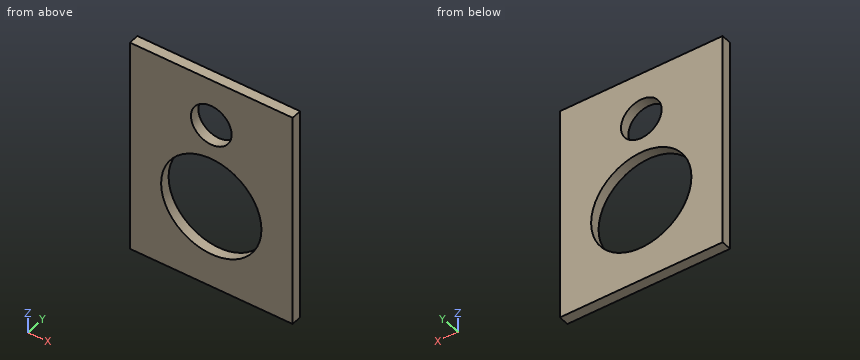
from build123d import *

# Parameters (mm, degrees)
F0_W     = 300
F0_H     = 400
F1_DEPTH = 19
F2_R     = 37.5
F2_R_2   = 92.5
F3_DEPTH = 19


with BuildPart() as f1:
    # F0 (on Front) → F1 (new body)
    with BuildSketch(Plane.XZ):
        with Locations((-9.787694, 40.103535)):
            Rectangle(F0_W, F0_H)
    extrude(amount=F1_DEPTH)

    # F2 (on face) → F3 (cut)
    with BuildSketch(Plane.XZ.offset(19)):
        with Locations((-9.787694, 152.603535)):
            Circle(F2_R)
        with Locations((-9.787694, -4.896465)):
            Circle(F2_R_2)
    extrude(amount=-F3_DEPTH, mode=Mode.SUBTRACT)


solid = f1.part
CAD build for the part. Positions are in the model's coordinates, mm. Give positions to 0.01 mm unless a question says otherwise; leave off trailing zeros. Order: outer loops, then holes, each group sorted by start corner. A loop starts at its lowest first (then second) coordinate and runs counter-clockwise, first axis right, second up. Notation, with made-up numbers: (0.25, 57) -> (55.25, 57) arc R20 cw to (55.25, 82) -> close; hole circle Ø9 at (88, 27.5). An arc over 180 degrees is marked (long way). Return JSON: item names as keys, results as strings.
Q1. Saw through at A-A (x = 46). Write the cut outline in (y, z).
Working result:
{"outline": "(-19, -159.9) -> (0, -159.9) -> (0, -78.68) -> (-19, -78.68) -> close; (-19, 68.89) -> (0, 68.89) -> (0, 240.1) -> (-19, 240.1) -> close"}
Q2. Saw through at C-C (y = -15). Write the cut outline in (x, z), then the cut area to 3 significant figures.
Working result:
{"outline": "(-159.79, -159.9) -> (140.21, -159.9) -> (140.21, 240.1) -> (-159.79, 240.1) -> close; hole circle Ø185 at (-9.79, -4.9); hole circle Ø75 at (-9.79, 152.6)", "area": "88,700 mm²"}
Q3. Drill centre lines: line 1 (Z direction, x = -37, y = -3); line 2 (X direction, y = -16.75, z = -3); line 3 (Z direction, x = -84.5, y = -16.25). Where is each one in solid material? Low to high.
Working result:
{"line 1": "-159.9 to -93.3, 83.51 to 126.8, 178.41 to 240.1", "line 2": "-159.79 to -102.27, 82.69 to 140.21", "line 3": "-159.9 to -59.43, 49.64 to 240.1"}
Q4. Saw through at B-B (z = 183). Write the cut outline in (x, y), then the cut area to 3 significant figures.
Working result:
{"outline": "(-159.79, -19) -> (-31.75, -19) -> (-31.75, 0) -> (-159.79, 0) -> close; (12.17, -19) -> (140.21, -19) -> (140.21, 0) -> (12.17, 0) -> close", "area": "4,870 mm²"}
